```python
from build123d import *

# Parameters (mm, degrees)
F0_R          = 5
F1_DEPTH      = 10.1
F2_R          = 4.8
F3_DEPTH      = 3
F5_DEPTH      = 5
F5_DEPTH_BACK = 57
F6_R          = 6
F7_DEPTH      = 3
F8_R          = 5
F9_DEPTH      = 30
F10_R         = 2.5
F11_DEPTH     = 80


with BuildPart() as f1:
    # F0 (on Right) → F1 (new body)
    with BuildSketch(Plane.YZ):
        Circle(F0_R)
    extrude(amount=-F1_DEPTH)

    # F2 (on face) → F3 (join)
    with BuildSketch(Plane.YZ):
        Circle(F2_R)
    extrude(amount=F3_DEPTH)

    # F4 (on face) → F5 (join, two sides)
    with BuildSketch(Plane.YZ.offset(3)) as f5_sk:
        Polygon((-4.565071, -1.483282), (0, -4.8), (4.565071, -1.483282), (2.821369, 3.883282), (-2.821369, 3.883282), align=None)
    extrude(amount=F5_DEPTH)
    extrude(f5_sk.sketch, amount=-F5_DEPTH_BACK)

    # F6 (on face) → F7 (join)
    with BuildSketch(Plane(origin=(-10.1, 0, 0), x_dir=(0, -1, 0), z_dir=(-1, 0, 0))):
        Circle(F6_R)
    extrude(amount=F7_DEPTH)

    # F8 (on face) → F9 (join)
    with BuildSketch(Plane(origin=(-13.1, 0, 0), x_dir=(0, -1, 0), z_dir=(-1, 0, 0))):
        Circle(F8_R)
    extrude(amount=F9_DEPTH)

    # F10 (on face) → F11 (cut)
    with BuildSketch(Plane.YZ.offset(8)):
        Circle(F10_R)
    extrude(amount=-F11_DEPTH, mode=Mode.SUBTRACT)


solid = f1.part
```
Geometry check sheet. Reference: the model listing, model coordinates, mm. A direction names the side the tool comes from. Round coordinates to 2 decimals unless told otherwise and drop trailing zeros. Write each loop counter-clockwise with the first axis right and the second up, starting at its lowest first coordinate (ties: lowest second). Pieces come first, ordered by that corner, then holes. Notation, with made-up numbers: (-39, 89) - (7, 89) arc R18 cw to (7, 107) - close; hole circle Ø6 at (36.25, 16.25). An arc over 180 degrees is marked (long way). Write each question's results on one line, items separated by ' | '.
(1) Set-up check for faces 1 (the face through (5.46, -3.68, 1.24)), 2 (the face through (5, 0, 3.883)), 3 (the face through (-13.1, 4, 4)), 4 (the face through (5.46, -2.31, -3.12)): record each of +Z, -Z, +X, -X, +Y, -Y from which the full face is reachable in a straight line by a thin tool's end or side.
Computed:
face 1: +Z, +X, -Y | face 2: +Z, +X, +Y, -Y | face 3: -X | face 4: -Z, +X, -Y
(2) Thickness scan on probe 1 along Z at (x, y) = (-41, 0); probe 2 along X at (y, z) = (2, -3.5); probe 3 along Z at (x, y) = (-36.5, -0.5). Record the ranges inside material, lowest first. Write a range as from..to.
Computed:
probe 1: z = -5..-2.5, 2.5..5 | probe 2: x = -43.1..3 | probe 3: z = -4.97..-2.45, 2.45..4.97
(3) Sectioned sample at B-B, the plane z = 0. Enter the section's corners in (x, y).
Computed:
outline: (-54, -4.08) - (-43.1, -4.08) - (-43.1, -5) - (-13.1, -5) - (-13.1, -6) - (-10.1, -6) - (-10.1, -5) - (0, -5) - (0, -4.8) - (3, -4.8) - (3, -4.08) - (8, -4.08) - (8, -2.5) - (-54, -2.5) - close; (-54, 2.5) - (8, 2.5) - (8, 4.08) - (3, 4.08) - (3, 4.8) - (0, 4.8) - (0, 5) - (-10.1, 5) - (-10.1, 6) - (-13.1, 6) - (-13.1, 5) - (-43.1, 5) - (-43.1, 4.08) - (-54, 4.08) - close
(4) Sectioned sample at C-C, the plane y = 3.5. Enter the section's corners in (x, z).
Computed:
outline: (-54, -2.26) - (-43.1, -2.26) - (-43.1, -3.57) - (-13.1, -3.57) - (-13.1, -4.87) - (-10.1, -4.87) - (-10.1, -3.57) - (0, -3.57) - (0, -3.28) - (3, -3.28) - (3, -2.26) - (8, -2.26) - (8, 1.79) - (3, 1.79) - (3, 3.28) - (0, 3.28) - (0, 3.57) - (-10.1, 3.57) - (-10.1, 4.87) - (-13.1, 4.87) - (-13.1, 3.57) - (-43.1, 3.57) - (-43.1, 1.79) - (-54, 1.79) - close
(5) Sectioned sample at A-A, the plane x = -44. Enter the section's corners in (y, z).
Computed:
outline: (-4.57, -1.48) - (0, -4.8) - (4.57, -1.48) - (2.82, 3.88) - (-2.82, 3.88) - close; hole circle Ø5 at (0, 0)
(6) Depth check by flat-ended pin: pin 1 Ø5 at (x, z) = (1.5, 0) entering from -Y; pin 2 Ø4.5 at (x, y) = (-49, -1) entering from +Z; pin 3 Ø1 at (x, z) = (-23.5, -4.5) entering from +Y. Enter the tip coordinate at first touch or a pass-through.
Computed:
pin 1: stops at y = -5 | pin 2: stops at z = 3.88 | pin 3: stops at y = 3
(7) Sectioned sample at D-D, the plane z = -3.5. Enter the section's corners in (x, y), plus the area to 3 significant figures.
Computed:
outline: (-54, -1.79) - (-43.1, -1.79) - (-43.1, -3.57) - (-13.1, -3.57) - (-13.1, -4.87) - (-10.1, -4.87) - (-10.1, -3.57) - (0, -3.57) - (0, -3.28) - (3, -3.28) - (3, -1.79) - (8, -1.79) - (8, 1.79) - (3, 1.79) - (3, 3.28) - (0, 3.28) - (0, 3.57) - (-10.1, 3.57) - (-10.1, 4.87) - (-13.1, 4.87) - (-13.1, 3.57) - (-43.1, 3.57) - (-43.1, 1.79) - (-54, 1.79) - close | area: 392 mm^2
